Source: CAD feature listing. Evaluate the final solid. Frame: model axes, mm. A direction names the side the tool comes from. Give positions to 0.01 mm unless a question says otherwise; leave off trailing zeros. Loops run counter-clockwise (first coordinate to the right, second up) from the corner with the lowest first, then second, coordinate; pieces in that order, holes last. Notation, with made-up numbers: (49, -23.5) -> (88, -23.5) arc R27 cw to (88, 0.5) -> close; hole circle Ø1 at (-7, 24). An arc over 180 degrees is marked (long way). Return JSON: item names as keys, results as strings. Group by question number.
(1) Access query for faces 5 (the face through (22, -27, 2.5)), 6 (the face through (2.96, -14.44, -2.46)), 7 (the face through (78, -26, -11)). Directions: +Z, -Z, +X, -X, +Y, -Y. A direction counts if a zero-diameter tool reaches every point of the face in a straight line with its end or side. Return the directions, or none.
(2) Cut plane D-D on x = 50. Return loops of the section in (y, z), then the cut area to 3 significant figures.
(3) Pin query (flat end, axial travel): pin 1 (2 mm diameter, centred on x = 54, y = -26.5, fed in from +Z); pin 2 (5 mm diameter, centred on x = 90, y = -6, fed in from +Z); pin 3 (7 mm diameter, centred on x = 47.5, y = -13, fed in from +Z); pin 4 (3 mm diameter, centred on x = 96.5, y = -4, fed in from -Z). Return the tip coordinate at first contact, or that it passes through.
(4) Draft query along Y for faces 1 (the face through (5.885, -3.249, -2.465)), 2 (the face through (94, -4, -2)), 3 (the face through (96, -26, -17)), 4 (the face through (5, -15, 0)). Return one class per face: released by +Y, released by -Y, zero draft, split by the parting line, or undercut.
(5) Cut plane B-B on z = -1.5. Give the number of separate pieces and of enclosed holes in the cut face, then the cut area to 3 significant figures.
(6) Cut plane C-C on z = -23. Return loops of the section in (x, y), then the cut area to 3 significant figures.
(7) Cut plane A-A on x = 3.5. Return loops of the section in (y, z).
(8) Ray query, line 1 (Y direction, x = 96.5, z = -2.1); line 2 (Y direction, x = 3, z = -2); line 3 (X direction, y = -4.5, z = -24). Return the intervals inside material, ascending. Write a range as from..to.
```python
from build123d import *

# Parameters (mm, degrees)
SKETCH3_W           = 100
SKETCH3_H           = 30
BOSS_EXTRUDE1_DEPTH = 30
SKETCH3_6_R         = 2.5
CUT_EXTRUDE1_DEPTH  = 25
CUT_EXTRUDE3_START  = -5
SKETCH3_9_W         = 7
SKETCH3_9_H         = 26
SKETCH3_9_R         = 2.5
CUT_EXTRUDE3_DEPTH  = 104.627804912
CUT_EXTRUDE4_DEPTH  = 2.5
BOSS_EXTRUDE2_DEPTH = 2.5
BOSS_EXTRUDE3_DEPTH = 5


with BuildPart() as part:
    # Sketch3 → Boss-Extrude1 (new body)
    with BuildSketch(Plane.XY):
        with Locations((50, -15)):
            Rectangle(SKETCH3_W, SKETCH3_H)
    extrude(amount=-BOSS_EXTRUDE1_DEPTH)

    # Sketch3_6 → Cut-Extrude1 (cut)
    with BuildSketch(Plane.XY):
        Polygon((35.214289751, 0), (8.952376915, 0), (9.860316922, -26), (34.306349745, -26), align=None)
        Polygon((61.880956418, 0), (38.119043582, 0), (39.026983589, -26), (60.973016411, -26), align=None)
        Polygon((91.047623085, 0), (64.785710249, 0), (65.693650255, -26), (90.139683078, -26), align=None)
        with Locations((3.5, -4)):
            Circle(SKETCH3_6_R)
        with Locations((3.5, -12)):
            Circle(SKETCH3_6_R)
        with Locations((3.5, -20)):
            Circle(SKETCH3_6_R)
        with Locations((96.5, -12)):
            Circle(SKETCH3_6_R)
        with Locations((96.5, -4)):
            Circle(SKETCH3_6_R)
        with Locations((96.5, -20)):
            Circle(SKETCH3_6_R)
    extrude(amount=-CUT_EXTRUDE1_DEPTH, mode=Mode.SUBTRACT)

    # Sketch3_9 → Cut-Extrude3 (cut, through all)
    # profile 1 of 8: a face of its own
    with BuildSketch(Plane.XY.offset(CUT_EXTRUDE3_START)):
        with Locations((3.5, -13)):
            Rectangle(SKETCH3_9_W, SKETCH3_9_H)
        with Locations((3.5, -20)):
            Circle(SKETCH3_9_R, mode=Mode.SUBTRACT)
        with Locations((3.5, -12)):
            Circle(SKETCH3_9_R, mode=Mode.SUBTRACT)
        with Locations((3.5, -4)):
            Circle(SKETCH3_9_R, mode=Mode.SUBTRACT)
    # profile 2 of 8: a face of its own
    with BuildSketch(Plane.XY.offset(CUT_EXTRUDE3_START)):
        with Locations((96.5, -13)):
            Rectangle(SKETCH3_9_W, SKETCH3_9_H)
        with Locations((96.5, -20)):
            Circle(SKETCH3_9_R, mode=Mode.SUBTRACT)
        with Locations((96.5, -12)):
            Circle(SKETCH3_9_R, mode=Mode.SUBTRACT)
        with Locations((96.5, -4)):
            Circle(SKETCH3_9_R, mode=Mode.SUBTRACT)
    # profile 3 of 8: a face of its own
    with BuildSketch(Plane.XY.offset(CUT_EXTRUDE3_START)):
        with Locations((3.5, -4)):
            Circle(SKETCH3_9_R)
    # profile 4 of 8: a face of its own
    with BuildSketch(Plane.XY.offset(CUT_EXTRUDE3_START)):
        with Locations((3.5, -12)):
            Circle(SKETCH3_9_R)
    # profile 5 of 8: a face of its own
    with BuildSketch(Plane.XY.offset(CUT_EXTRUDE3_START)):
        with Locations((3.5, -20)):
            Circle(SKETCH3_9_R)
    # profile 6 of 8: a face of its own
    with BuildSketch(Plane.XY.offset(CUT_EXTRUDE3_START)):
        with Locations((96.5, -20)):
            Circle(SKETCH3_9_R)
    # profile 7 of 8: a face of its own
    with BuildSketch(Plane.XY.offset(CUT_EXTRUDE3_START)):
        with Locations((96.5, -4)):
            Circle(SKETCH3_9_R)
    # profile 8 of 8: a face of its own
    with BuildSketch(Plane.XY.offset(CUT_EXTRUDE3_START)):
        with Locations((96.5, -12)):
            Circle(SKETCH3_9_R)
    extrude(amount=-CUT_EXTRUDE3_DEPTH, mode=Mode.SUBTRACT)

    # Sketch3_10 → Cut-Extrude4 (cut)
    with BuildSketch(Plane.XY):
        Polygon((34.236508206, -28), (9.930158461, -28), (10, -30), (34.166666667, -30), align=None)
        Polygon((60.903174872, -28), (39.096825128, -28), (39.166666667, -30), (60.833333333, -30), align=None)
        Polygon((90.069841539, -28), (65.763491794, -28), (65.833333333, -30), (90, -30), align=None)
    extrude(amount=-CUT_EXTRUDE4_DEPTH, mode=Mode.SUBTRACT)

    # Sketch3_11 → Boss-Extrude2 (add)
    with BuildSketch(Plane.XY):
        Polygon((34.306349745, -26), (9.860316922, -26), (9.930158461, -28), (34.236508206, -28), align=None)
        Polygon((60.973016411, -26), (39.026983589, -26), (39.096825128, -28), (60.903174872, -28), align=None)
        Polygon((90.139683078, -26), (65.693650255, -26), (65.763491794, -28), (90.069841539, -28), align=None)
    extrude(amount=BOSS_EXTRUDE2_DEPTH)

    # Sketch3_12 → Boss-Extrude3 (add)
    with BuildSketch(Plane.XY):
        Polygon((37.118434038, 0), (36.214899296, 0), (35.306959289, -26), (38.026374044, -26), align=None)
        Polygon((38.026374044, -26), (35.306959289, -26), (35.23711775, -28), (38.096215583, -28), align=None)
        Polygon((38.096215583, -28), (35.23711775, -28), (35.167276211, -30), (38.166057122, -30), align=None)
        Polygon((64.76288225, -28), (61.903784417, -28), (61.833942878, -30), (64.832723789, -30), align=None)
        Polygon((64.693040711, -26), (61.973625956, -26), (61.903784417, -28), (64.76288225, -28), align=None)
        Polygon((63.785100704, 0), (62.881565962, 0), (61.973625956, -26), (64.693040711, -26), align=None)
    extrude(amount=BOSS_EXTRUDE3_DEPTH)


solid = part.part
```
Answers:
{
 "1": {"face 5": "+Z, -X, +Y, -Y", "face 6": "+Z, -Z", "face 7": "+Z, +Y"},
 "2": {"outline": "(-30, -30) -> (0, -30) -> (0, -25) -> (-26, -25) -> (-26, 2.5) -> (-28, 2.5) -> (-28, -2.5) -> (-30, -2.5) -> close", "area": "250 mm²"},
 "3": {"pin 1": "z = 2.5", "pin 2": "z = 0", "pin 3": "z = -25", "pin 4": "through"},
 "4": {"face 1": "undercut", "face 2": "undercut", "face 3": "released by +Y", "face 4": "zero draft"},
 "5": {"separate pieces": "1", "enclosed holes": "6", "area": "829 mm²"},
 "6": {"outline": "(0, -30) -> (100, -30) -> (100, -26) -> (93, -26) -> (93, 0) -> (91.05, 0) -> (90.14, -26) -> (65.69, -26) -> (64.79, 0) -> (61.88, 0) -> (60.97, -26) -> (39.03, -26) -> (38.12, 0) -> (35.21, 0) -> (34.31, -26) -> (9.86, -26) -> (8.95, 0) -> (7, 0) -> (7, -26) -> (0, -26) -> close", "area": "723 mm²"},
 "7": {"outline": "(-30, -30) -> (-26, -30) -> (-26, -5) -> (-22.5, -5) -> (-22.5, 0) -> (-30, 0) -> close; (-17.5, -5) -> (-14.5, -5) -> (-14.5, 0) -> (-17.5, 0) -> close; (-9.5, -5) -> (-6.5, -5) -> (-6.5, 0) -> (-9.5, 0) -> close; (-1.5, -5) -> (0, -5) -> (0, 0) -> (-1.5, 0) -> close"},
 "8": {"line 1": "-30..-22.5, -17.5..-14.5, -9.5..-6.5, -1.5..0", "line 2": "-30..-22.45, -17.55..-14.45, -9.55..-6.45, -1.55..0", "line 3": "7..9.11, 35.06..38.28, 61.72..64.94, 90.89..93"}
}
